```python
from build123d import *

# Parameters (mm, degrees)
SKETCH1_R           = 16
SKETCH1_R_2         = 12.7
BOSS_EXTRUDE1_DEPTH = 40
SKETCH2_R           = 16
BOSS_EXTRUDE2_DEPTH = 10
BOSS_EXTRUDE3_DEPTH = 20
CUT_EXTRUDE1_DEPTH  = 5


with BuildPart() as part:
    # Sketch1 → Boss-Extrude1 (new body)
    with BuildSketch(Plane(origin=(0, 0, 0), x_dir=(1, 0, 0), z_dir=(0, 1, 0))):
        with Locations(Location((0, 0, 0), (0, 0, 270))):
            Circle(SKETCH1_R)
        with Locations(Location((0, 0, 0), (0, 0, 270))):
            Circle(SKETCH1_R_2, mode=Mode.SUBTRACT)
    extrude(amount=BOSS_EXTRUDE1_DEPTH)

    # Sketch2 → Boss-Extrude2 (add)
    with BuildSketch(Plane(origin=(0, 40, 0), x_dir=(1, 0, 0), z_dir=(0, 1, 0))):
        with Locations(Location((0, 0, 0), (0, 0, 270))):
            Circle(SKETCH2_R)
    extrude(amount=BOSS_EXTRUDE2_DEPTH)

    # Sketch3 → Boss-Extrude3 (add)
    with BuildSketch(Plane(origin=(0, 50, 0), x_dir=(1, 0, 0), z_dir=(0, 1, 0))):
        Polygon((0, -10), (0, 0), (0, 10), (-2.5, 10), (-2.5, -10), align=None)
        Polygon((0, 10), (0, 0), (0, -10), (2.5, -10), (2.5, 10), align=None)
    extrude(amount=BOSS_EXTRUDE3_DEPTH)

    # Sketch4 → Cut-Extrude1 (cut)
    with BuildSketch(Plane(origin=(2.5, 0, 0), x_dir=(0, 0, -1), z_dir=(1, 0, 0))):
        with BuildLine():
            Line((0, 70), (-10, 70))
            Line((-10, 70), (-10, 60))
            ThreePointArc((-10, 60), (-7.071067812, 67.071067812), (0, 70))
        make_face()
        with BuildLine():
            Line((10, 70), (0, 70))
            ThreePointArc((0, 70), (7.071067812, 67.071067812), (10, 60))
            Line((10, 60), (10, 70))
        make_face()
        with BuildLine():
            ThreePointArc((2, 60), (1.414213562, 61.414213562), (0, 62))
            Line((0, 62), (0, 58))
            ThreePointArc((0, 58), (1.414213562, 58.585786438), (2, 60))
        make_face()
        with BuildLine():
            Line((0, 58), (0, 62))
            ThreePointArc((0, 62), (-2, 60), (0, 58))
        make_face()
    extrude(amount=-CUT_EXTRUDE1_DEPTH, mode=Mode.SUBTRACT)


solid = part.part
```
Here's how the part is built. I have some questions about the finished solid (model axes, mm). A direction names the side the tool comes from. Round coordinates to 2 decimals unless told otherwise and drop trailing zeros. Loops run counter-clockwise (first coordinate to the right, second up) from the corner with the lowest first, then second, coordinate; pieces in that order, holes last. Notation, with made-up numbers: (-33, 16) -> (-8, 16) arc R20 ccw to (-8, 23) -> close; hole circle Ø6 at (58.5, 17.5). An arc over 180 degrees is marked (long way). Answer as CSV lines item,"result". Start each with the question number.
1. Imagine slicing it at C-C on z = -6.5. Write out the boundary of the cut face in (x, y).
2. I need wall thicknesses on probe 1 along X at (y, z) = (18, 0); probe 2 along Y at (x, z) = (-3.5, 12.5); probe 3 along Y at (x, z) = (-7, -10.5). Which ranges of each line are inside material? Lowest first, please. Write a range as from..to.
3. Imagine slicing it at D-D on x = -4.5. Write out the boundary of the cut face in (y, z), plus the area to 3 significant figures.
4. I'm going to push flat-ended pins straight in: P1, Ø2, axis at y = 38, z = 7, coming from the +X side; P2, Ø5, axis at x = 2.5, z = -11, coming from the +Y side; P3, Ø16, axis at x = -3.5, z = 1.5, coming from the +Y side; P4, Ø2, axis at x = -8.5, z = 2.5, coming from the +Y side. Where does each tip first touch, or does it pass through?
5. Imagine slicing it at A-A on x = 0. Write out the boundary of the cut face in (y, z), plus the area to 3 significant figures.
6. If we mould it in two halves opening along Z, with no side actions, what happens to faces 1 (the face through (2.5, 57.6, 0.1)), 2 (the face through (0, 55, -10)), 3 (the face through (0, 40, 0))? For each: pulls with the +Z half, pulls with the -Z half, needs draft (parallel to the pull), parting line crosses it, or undercut.
7. For faces 4 (the face through (0, 55, 10)), 5 (the face through (-2.5, 57.6, -0.1)), 6 (the face through (12, 0, -5)), 7 (the face through (-7.7, 19.7, -10.1)), 8 (the face through (-15.62, 24.65, -3.47)), which set-ups out of +Z, -Z, +X, -X, +Y, -Y let a thin tool reach every point of the face, with its end or its side?
8. Imagine slicing it at B-B on y = 19. Write out the boundary of the cut face in (x, z).
Solution:
1,outline,"(-14.62, 0) -> (-10.91, 0) -> (-10.91, 40) -> (10.91, 40) -> (10.91, 0) -> (14.62, 0) -> (14.62, 50) -> (2.5, 50) -> (2.5, 67.6) -> (-2.5, 67.6) -> (-2.5, 50) -> (-14.62, 50) -> close"
2,probe 1,"-16..-12.7, 12.7..16"
2,probe 2,"0..50"
2,probe 3,"40..50"
3,outline,"(0, -15.35) -> (50, -15.35) -> (50, 15.35) -> (0, 15.35) -> (0, 11.88) -> (40, 11.88) -> (40, -11.88) -> (0, -11.88) -> close"
3,area,"585 mm²"
4,P1,"x = 14.83"
4,P2,"y = 65.27"
4,P3,"y = 70"
4,P4,"y = 50"
5,outline,"(0, -16) -> (50, -16) -> (50, -10) -> (60, -10) arc R10 ccw to (60, 10) -> (50, 10) -> (50, 16) -> (0, 16) -> (0, 12.7) -> (40, 12.7) -> (40, -12.7) -> (0, -12.7) -> close; hole circle Ø4 at (60, 0)"
5,area,"929 mm²"
6,face 1,"needs draft"
6,face 2,"pulls with the -Z half"
6,face 3,"undercut"
7,face 4,"+Z, +X, -X, +Y"
7,face 5,"+Z, -Z, -X, +Y"
7,face 6,"+Z, -Z, +X, -X, -Y"
7,face 7,"-Y"
7,face 8,"+Y, -Y"
8,outline,"circle Ø32 at (0, 0); hole circle Ø25.4 at (0, 0)"
